Design review of the part built by this model. Coordinates are the model's own, in mm. Coordinates: 2 decimals unless noted, no trailing zeros. Order: outer loops, then holes, each group sorted by start corner. A loop starts at its lowest first (then second) coordinate and runs counter-clockwise, first axis right, second up. Notation, with made-up numbers: (35.5, 8) -> (70.5, 8) arc R21 ccw to (70.5, 16) -> close; hole circle Ø2 at (-3.75, 39.25). An arc over 180 degrees is marked (long way). Write item = value, one per line.
```python
from build123d import *

# Parameters (mm, degrees)
SKETCH1_W           = 53.515278819
SKETCH1_H           = 1.25
BOSS_EXTRUDE1_DEPTH = 0.65
SKETCH2_R           = 1.6
CUT_EXTRUDE1_DEPTH  = 41.32396752


with BuildPart() as part:
    # Sketch1 → Boss-Extrude1 (new body)
    with BuildSketch(Plane(origin=(0, 0, 0), x_dir=(1, 0, 0), z_dir=(0, 1, 0))):
        Polygon((-27.428763177, -6.643775098), (-27.428763177, 29.222168516), (-27.428763177, 29.551020407), (26.086515642, 29.551020407), (26.086515642, 28.356224902), (26.086515642, -6.643775098), align=None)
        with Locations((-0.671123767, -7.268775098)):
            Rectangle(SKETCH1_W, SKETCH1_H)
    extrude(amount=BOSS_EXTRUDE1_DEPTH)

    # Sketch2 → Cut-Extrude1 (cut, through all)
    with BuildSketch(Plane.XZ):
        with Locations(Location((-20.106484358, -11.691224902, 0), (0, 0, 270))):
            Circle(SKETCH2_R)
        with Locations(Location((17.882515642, -24.493824902, 0), (0, 0, 270))):
            Circle(SKETCH2_R)
        with Locations(Location((17.882515642, 3.040775098, 0), (0, 0, 270))):
            Circle(SKETCH2_R)
    extrude(amount=-CUT_EXTRUDE1_DEPTH, mode=Mode.SUBTRACT)


solid = part.part
```
(1) For L1, parallel to Z at x = -20, y = 0.2; L2, parallel to X at y = 0.3, z = 4.5; L3, parallel to X at y = 0.4, z = -25, list the stretches that pass through material, from the lowest coordinate up.
Report:
L1 = -29.55 to -13.29, -10.09 to 7.89
L2 = -27.43 to 17.23, 18.54 to 26.09
L3 = -27.43 to 16.36, 19.4 to 26.09
(2) The part is to be moulded in two halves that separate along X. For faces 1 (the cylindrical face through (-18.757, 0.32, -12.551)), 2 (the flat face through (0, 0.65, -11)), say which applies: released by +X, released by -X, zero draft, split by the parting line, or undercut.
Report:
face_1 = undercut
face_2 = zero draft
(3) We need section A-A (z = -12.5). Write out the cut boundary in (x, y), and give its area (3 significant figures).
Report:
outline = (-27.43, 0) -> (-21.49, 0) -> (-21.49, 0.65) -> (-27.43, 0.65) -> close; (-18.73, 0) -> (26.09, 0) -> (26.09, 0.65) -> (-18.73, 0.65) -> close
area = 33.0 mm²
